For this review, take the finished solid that the model builds, in its own axes (mm). A direction names the side the tool comes from. Give positions to 0.01 mm unless a question says otherwise; leave off trailing zeros. Loops run counter-clockwise (first coordinate to the right, second up) from the corner with the lowest first, then second, coordinate; pieces in that order, holes last.
```python
from build123d import *

# Parameters (mm, degrees)
SKETCH1_W               = 60
SKETCH1_H               = 130
BOSS_EXTRUDE1_DEPTH     = 40
SKETCH2_R               = 28.25
SKETCH2_R_2             = 13.25
SKETCH2_R_3             = 17.25
SKETCH2_R_4             = 6.75
SKETCH2_R_5             = 9.5
CUT_EXTRUDE1_DEPTH      = 38
CUT_EXTRUDE9_DEPTH      = 83.006097334
CUT_EXTRUDE9_DEPTH_BACK = 83.006097334
CUT_EXTRUDE10_START     = 2
CUT_EXTRUDE10_DEPTH     = 81.006097334
CUT_EXTRUDE11_REACH     = 99.082
FILLET8_R               = 5
FILLET9_R               = 10
FILLET10_R              = 2.5
FILLET11_R              = 5


with BuildPart() as part:
    # Sketch1 → Boss-Extrude1 (new body)
    with BuildSketch(Plane(origin=(0, 0, 0), x_dir=(0, 1, 0), z_dir=(0, 0, 1))):
        Rectangle(SKETCH1_W, SKETCH1_H)
    extrude(amount=BOSS_EXTRUDE1_DEPTH)

    # Sketch2 → Cut-Extrude1 (cut)
    with BuildSketch(Plane.XY.offset(40)):
        with Locations((-35, 0)):
            Circle(SKETCH2_R)
        with Locations((37, -14.75)):
            Circle(SKETCH2_R_2)
        with Locations((12, 10.75)):
            Circle(SKETCH2_R_3)
        with Locations((56.25, 21.25)):
            Circle(SKETCH2_R_4)
        with Locations((42, 10)):
            Circle(SKETCH2_R_5)
        with BuildLine():
            Line((63, -5), (63, -25))
            ThreePointArc((63, -25), (60, -28), (57, -25))
            Line((57, -25), (57, -5))
            ThreePointArc((57, -5), (60, -2), (63, -5))
        make_face()
    extrude(amount=-CUT_EXTRUDE1_DEPTH, mode=Mode.SUBTRACT)

    # Sketch11 → Cut-Extrude9 (cut, two sides: drawn at the far end of the back side and taken through both)
    with BuildSketch(Plane(origin=(0, 0, 0), x_dir=(-1, 0, 0), z_dir=(0, 1, 0)).offset(-CUT_EXTRUDE9_DEPTH_BACK)):
        Polygon((37.662617959, 40), (-65, 40), (-65, 22.5), (-33.857500095, 22.5), (-14.42300462, 27), (19.914447088, 27), align=None)
    extrude(amount=CUT_EXTRUDE9_DEPTH + CUT_EXTRUDE9_DEPTH_BACK, mode=Mode.SUBTRACT)

    # Sketch12 → Cut-Extrude10 (cut, through all)
    with BuildSketch(Plane(origin=(0, 0, 0), x_dir=(0, 1, 0), z_dir=(0, 0, 1)).offset(CUT_EXTRUDE10_START)):
        with BuildLine():
            Line((-25.153127982, 19.113444278), (-28, 19.113444278))
            Line((-28, 19.113444278), (-28, -14.42300462))
            Line((-28, -14.42300462), (-28, -30.519259302))
            ThreePointArc((-28, -30.519259302), (-21.630520462, -23.953125349), (-12.614481333, -22.405409906))
            Line((-12.614481333, -22.405409906), (-7.568879853, -15.997641924))
            ThreePointArc((-7.568879853, -15.997641924), (-7.137176738, -6.377597635), (-1.98737408, 1.759425917))
            Line((-1.98737408, 1.759425917), (-5.735279815, 5.808065062))
            ThreePointArc((-5.735279815, 5.808065062), (-16.816114685, 10.458590364), (-25.153127982, 19.113444278))
        make_face()
    extrude(amount=CUT_EXTRUDE10_DEPTH, mode=Mode.SUBTRACT)

    # Sketch13 → Cut-Extrude11 (cut, up to next)
    with BuildSketch(Plane.XZ.offset(30), mode=Mode.PRIVATE) as cut_extrude11_sk1:
        Polygon((-15.112535459, 27), (35.351266766, 27), (6.364131369, 5), (-6.135868631, 5), align=None)
    cut_extrude11_tool1 = extrude(cut_extrude11_sk1.sketch, amount=-CUT_EXTRUDE11_REACH, mode=Mode.PRIVATE) & part.part
    add(cut_extrude11_tool1.solids().sort_by_distance((6.122185, -30, 18.210804))[0], mode=Mode.SUBTRACT)

    # Fillet8
    fillet8_edges = [part.edges().sort_by_distance(p)[0] for p in [
        (65, 30, 11.25),
        (65, -30, 11.25),
        (-65, -30, 20),
        (-65, 30, 20),
    ]]
    fillet(fillet8_edges, radius=FILLET8_R)

    # Fillet9
    # the kernel refuses this fillet: 10 mm, written as the material it adds along each edge
    with BuildSketch(Plane(origin=(33.857500095, -30, 22.5), x_dir=(1, 0, 0), z_dir=(0, 1, 0))) as fillet9_piece_1_section:
        with BuildLine():
            CenterArc((FILLET9_R * 0.114262005899, -FILLET9_R), FILLET9_R, 90, 13.036921742)
            Line((-FILLET9_R * 0.111316891577, -FILLET9_R * 0.0257750973141), (0, 0))
            Line((0, 0), (FILLET9_R * 0.114262005899, 0))
        make_face()
    fillet9_piece_1 = extrude(amount=5.234596359, mode=Mode.PRIVATE)
    fillet9_piece_1 = fillet9_piece_1 - Plane(origin=(37, -14.75, 22.477974756), x_dir=(1, 0, 0), z_dir=(0, 0, 1)) * Cylinder(13.25, 16, mode=Mode.PRIVATE)
    add(fillet9_piece_1)
    with BuildSketch(Plane(origin=(33.857500095, -4.734596359, 22.5), x_dir=(1, 0, 0), z_dir=(0, 1, 0))) as fillet9_piece_2_section:
        with BuildLine():
            CenterArc((FILLET9_R * 0.114262005899, -FILLET9_R), FILLET9_R, 90, 13.036921742)
            Line((-FILLET9_R * 0.111316891577, -FILLET9_R * 0.0257750973141), (0, 0))
            Line((0, 0), (FILLET9_R * 0.114262005899, 0))
        make_face()
    fillet9_piece_2 = extrude(amount=12.697303917, mode=Mode.PRIVATE)
    fillet9_piece_2 = fillet9_piece_2 - Plane(origin=(37, -14.75, 22.48681781), x_dir=(1, 0, 0), z_dir=(0, 0, 1)) * Cylinder(13.25, 30, mode=Mode.PRIVATE)
    fillet9_piece_2 = fillet9_piece_2 - Plane(origin=(42, 10, 22.48681781), x_dir=(1, 0, 0), z_dir=(0, 0, 1)) * Cylinder(9.5, 30, mode=Mode.PRIVATE)
    add(fillet9_piece_2)
    with BuildSketch(Plane(origin=(33.857500095, 12.037292442, 22.5), x_dir=(1, 0, 0), z_dir=(0, 1, 0))) as fillet9_piece_3_section:
        with BuildLine():
            CenterArc((FILLET9_R * 0.114262005899, -FILLET9_R), FILLET9_R, 90, 13.036921742)
            Line((-FILLET9_R * 0.111316891577, -FILLET9_R * 0.0257750973141), (0, 0))
            Line((0, 0), (FILLET9_R * 0.114262005899, 0))
        make_face()
    fillet9_piece_3 = extrude(amount=17.962707558, mode=Mode.PRIVATE)
    fillet9_piece_3 = fillet9_piece_3 - Plane(origin=(42, 10, 22.478816229), x_dir=(1, 0, 0), z_dir=(0, 0, 1)) * Cylinder(9.5, 41, mode=Mode.PRIVATE)
    add(fillet9_piece_3)
    with BuildSketch(Plane(origin=(-19.914447088, -15.708414802, 27), x_dir=(1, 0, 0), z_dir=(0, -1, 0))) as fillet9_piece_4_section:
        with BuildLine():
            CenterArc((FILLET9_R * 0.327059529607, FILLET9_R), FILLET9_R, 233.778347997, 36.221652003)
            Line((-FILLET9_R * 0.263851045123, FILLET9_R * 0.193262934611), (0, 0))
            Line((0, 0), (FILLET9_R * 0.327059529607, 0))
        make_face()
    fillet9_piece_4 = extrude(amount=14.291585198, mode=Mode.PRIVATE)
    fillet9_piece_4 = fillet9_piece_4 & Plane(origin=(-35, 0, 26.964300655), x_dir=(0.9812415105326922, -0.19278251478679478, 0), z_dir=(0, 0, -1)) * Cylinder(29.75, 42, mode=Mode.PRIVATE)
    fillet9_piece_4 = split(fillet9_piece_4, bisect_by=Plane(origin=(-19.113444278, -23.524724426, 26.964300655), z_dir=(1, 0, 0)), keep=Keep.TOP, mode=Mode.PRIVATE)
    fillet9_piece_4 = fillet9_piece_4 - Plane(origin=(-35, 0, 26.964300655), x_dir=(1, 0, 0), z_dir=(0, 0, 1)) * Cylinder(28.25, 42, mode=Mode.PRIVATE)
    add(fillet9_piece_4)
    with BuildSketch(Plane(origin=(-19.914447088, -15.708414802, 27), x_dir=(1, 0, 0), z_dir=(0, -1, 0))) as fillet9_piece_5_section:
        with BuildLine():
            CenterArc((FILLET9_R * 0.327059529607, FILLET9_R), FILLET9_R, 233.778347997, 36.221652003)
            Line((-FILLET9_R * 0.263851045123, FILLET9_R * 0.193262934611), (0, 0))
            Line((0, 0), (FILLET9_R * 0.327059529607, 0))
        make_face()
    fillet9_piece_5 = extrude(amount=14.291585198, mode=Mode.PRIVATE)
    fillet9_piece_5 = fillet9_piece_5 & Plane(origin=(-35, 0, 27.570308722), x_dir=(0.9812415105326922, -0.19278251478679478, 0), z_dir=(0, 0, -1)) * Cylinder(29.75, 42, mode=Mode.PRIVATE)
    fillet9_piece_5 = split(fillet9_piece_5, bisect_by=Plane(origin=(-19.113444278, -25.104682391, 27.570308722), z_dir=(-1, 0, 0)), keep=Keep.TOP, mode=Mode.PRIVATE)
    fillet9_piece_5 = fillet9_piece_5 - Plane(origin=(-35, 0, 27.570308722), x_dir=(1, 0, 0), z_dir=(0, 0, 1)) * Cylinder(28.25, 42, mode=Mode.PRIVATE)
    add(fillet9_piece_5)
    with BuildSketch(Plane(origin=(-19.914447088, -15.708414802, 27), x_dir=(1, 0, 0), z_dir=(0, -1, 0))) as fillet9_piece_6_section:
        with BuildLine():
            CenterArc((FILLET9_R * 0.327059529607, FILLET9_R), FILLET9_R, 233.778347997, 36.221652003)
            Line((-FILLET9_R * 0.263851045123, FILLET9_R * 0.193262934611), (0, 0))
            Line((0, 0), (FILLET9_R * 0.327059529607, 0))
        make_face()
    fillet9_piece_6 = extrude(amount=14.291585198, mode=Mode.PRIVATE)
    fillet9_piece_6 = fillet9_piece_6 - Plane(origin=(-35, 0, 27.459351012), x_dir=(0.9812415105326922, -0.19278251478679478, 0), z_dir=(0, 0, -1)) * Cylinder(29.75, 42, mode=Mode.PRIVATE)
    fillet9_piece_6 = split(fillet9_piece_6, bisect_by=Plane(origin=(-19.113444278, -26.928061773, 27.459351012), z_dir=(-1, 0, 0)), keep=Keep.TOP, mode=Mode.PRIVATE)
    fillet9_piece_6 = split(fillet9_piece_6, bisect_by=Plane(origin=(-20.316684316, -28, 27.459351012), z_dir=(0, 1, 0)), keep=Keep.TOP, mode=Mode.PRIVATE)
    add(fillet9_piece_6)
    with BuildSketch(Plane(origin=(-19.914447088, -15.708414802, 27), x_dir=(1, 0, 0), z_dir=(0, -1, 0))) as fillet9_piece_7_section:
        with BuildLine():
            CenterArc((FILLET9_R * 0.327059529607, FILLET9_R), FILLET9_R, 233.778347997, 36.221652003)
            Line((-FILLET9_R * 0.263851045123, FILLET9_R * 0.193262934611), (0, 0))
            Line((0, 0), (FILLET9_R * 0.327059529607, 0))
        make_face()
    fillet9_piece_7 = extrude(amount=14.291585198, mode=Mode.PRIVATE)
    fillet9_piece_7 = split(fillet9_piece_7, bisect_by=Plane(origin=(-19.113444278, -29, 26.965326642), z_dir=(1, 0, 0)), keep=Keep.TOP, mode=Mode.PRIVATE)
    fillet9_piece_7 = split(fillet9_piece_7, bisect_by=Plane(origin=(-18.088636338, -28, 26.965326642), z_dir=(0, -1, 0)), keep=Keep.TOP, mode=Mode.PRIVATE)
    add(fillet9_piece_7)
    with BuildSketch(Plane(origin=(-19.914447088, -15.708414802, 27), x_dir=(1, 0, 0), z_dir=(0, -1, 0))) as fillet9_piece_8_section:
        with BuildLine():
            CenterArc((FILLET9_R * 0.327059529607, FILLET9_R), FILLET9_R, 233.778347997, 36.221652003)
            Line((-FILLET9_R * 0.263851045123, FILLET9_R * 0.193262934611), (0, 0))
            Line((0, 0), (FILLET9_R * 0.327059529607, 0))
        make_face()
    fillet9_piece_8 = extrude(amount=14.291585198, mode=Mode.PRIVATE)
    fillet9_piece_8 = split(fillet9_piece_8, bisect_by=Plane(origin=(-19.113444278, -29, 27.580257853), z_dir=(-1, 0, 0)), keep=Keep.TOP, mode=Mode.PRIVATE)
    fillet9_piece_8 = split(fillet9_piece_8, bisect_by=Plane(origin=(-20.54645477, -28, 27.580257853), z_dir=(0, -1, 0)), keep=Keep.TOP, mode=Mode.PRIVATE)
    add(fillet9_piece_8)
    with BuildSketch(Plane(origin=(-19.914447088, 30, 27), x_dir=(-0.8067370653888534, 0, 0.5909105747300355), z_dir=(0, -1, 0))) as fillet9_piece_9_section:
        with BuildLine():
            CenterArc((FILLET9_R * 0.327059529607, -FILLET9_R), FILLET9_R, 90, 36.221652003)
            Line((-FILLET9_R * 0.263851045123, -FILLET9_R * 0.193262934611), (0, 0))
            Line((0, 0), (FILLET9_R * 0.327059529607, 0))
        make_face()
    fillet9_piece_9 = extrude(amount=14.291585198, mode=Mode.PRIVATE)
    fillet9_piece_9 = fillet9_piece_9 - Plane(origin=(-35, 0, 27.325753935), x_dir=(1, 0, 0), z_dir=(0, 0, 1)) * Cylinder(28.25, 42, mode=Mode.PRIVATE)
    add(fillet9_piece_9)
    # the kernel refuses this fillet: 10 mm, written as the material it takes off along each edge
    with BuildSketch(Plane(origin=(14.42300462, 32.856550147, 27), x_dir=(0.9742249026859169, 0, -0.22557889747628432), z_dir=(0, -1, 0))) as fillet9_2_piece_1:
        with BuildLine():
            CenterArc((FILLET9_R * 0.114262005899, -FILLET9_R), FILLET9_R, 90, 13.036921742)
            Line((-FILLET9_R * 0.111316891577, -FILLET9_R * 0.0257750973141), (0, 0))
            Line((0, 0), (FILLET9_R * 0.114262005899, 0))
        make_face()
    extrude(amount=7.884120565, mode=Mode.SUBTRACT)
    with BuildSketch(Plane(origin=(14.42300462, -3.472429582, 27), x_dir=(0.9742249026859169, 0, -0.22557889747628432), z_dir=(0, -1, 0))) as fillet9_2_piece_2:
        with BuildLine():
            CenterArc((FILLET9_R * 0.114262005899, -FILLET9_R), FILLET9_R, 90, 13.036921742)
            Line((-FILLET9_R * 0.111316891577, -FILLET9_R * 0.0257750973141), (0, 0))
            Line((0, 0), (FILLET9_R * 0.114262005899, 0))
        make_face()
    extrude(amount=7.226902729, mode=Mode.SUBTRACT)
    with BuildSketch(Plane(origin=(-37.662617959, 38.17648824, 40), x_dir=(0.8067370653888553, 0, -0.5909105747300331), z_dir=(0, -1, 0)), Plane(origin=(-37.662617959, -19.94775336, 40), x_dir=(0.8067370653888553, 0, -0.5909105747300331), z_dir=(0, -1, 0))) as fillet9_2_piece_3:
        with BuildLine():
            CenterArc((FILLET9_R * 0.327059529607, -FILLET9_R), FILLET9_R, 90, 36.221652003)
            Line((-FILLET9_R * 0.263851045123, -FILLET9_R * 0.193262934611), (0, 0))
            Line((0, 0), (FILLET9_R * 0.327059529607, 0))
        make_face()
    extrude(amount=18.22873488, mode=Mode.SUBTRACT)

    # Fillet10
    fillet10_edges = [part.edges().sort_by_distance(p)[0] for p in [
        (22.405409906, -12.614481333, 13.575848822),
        (15.997641924, -7.568879853, 14.317698693),
        (-1.759425917, -1.98737408, 14.5),
        (-5.808065062, -5.735279815, 14.5),
    ]]
    fillet(fillet10_edges, radius=FILLET10_R)

    # Fillet11
    fillet11_edges = [part.edges().sort_by_distance(p)[0] for p in [
        (6.364131369, -29, 5),
        (-6.135868631, -29, 5),
        (-15.112535459, -29, 27),
    ]]
    fillet(fillet11_edges, radius=FILLET11_R)


solid = part.part
```
Q1. Machinability: for faces 1 (the cylindrical face through (64, 28, 11)), 2 (the cylindrical face through (-63.223, 1.242, 17.044)), which of the approach directions +Z, -Z, +X, -X, +Y, -Y give a long, thin tool a straight path to every point of the face, cutting with its end or side? Answer none if there is none.
Answers:
face 1: +Z, -Z, +X, +Y
face 2: +Z
Q2. Consider section B-B on x = 6.5. Give the boundary of the cut face in (y, z), plus the area to 3 significant figures.
Answers:
outline: (-30, 0) - (30, 0) - (30, 27) - (27.1, 27) - (27.1, 2) - (-5.6, 2) - (-5.6, 27) - (-7.18, 27) - (-7.18, 2) - (-28, 2) - (-28, 5.34) - (-30, 5.34) - close
area: 239 mm2
Q3. For pin 1 Ø9 at (x, y) = (47, 12.5) entering from +Z; pin 2 Ø8 at (x, y) = (41, -9) entering from +Z; pin 3 Ø21 at (x, y) = (44, 12.5) entering from +Z, all flat-tipped, find the tip position at first contact; note any pin that passes through.
Answers:
pin 1: stops at z = 22.5
pin 2: stops at z = 2
pin 3: stops at z = 22.58
Q4. Consider section D-D on y = -16. Give the boundary of the cut face in (x, z).
Answers:
outline: (-65, 0) - (65, 0) - (65, 22.5) - (63, 22.5) - (63, 2) - (57, 2) - (57, 22.5) - (50.19, 22.5) - (50.19, 2) - (23.81, 2) - (23.81, 24.83) - (22.3, 25.18) - (22.3, 2) - (-9.92, 2) - (-9.92, 27) - (-11.72, 27) - (-11.72, 2) - (-58.28, 2) - (-58.28, 40) - (-65, 40) - close
Q5. Consider section A-A on y = 2. Give the boundary of the cut face in (x, z), plus the area to 3 significant figures.
Answers:
outline: (-65, 0) - (65, 0) - (65, 22.5) - (47.12, 22.5) - (47.12, 2) - (36.88, 2) - (36.88, 22.5) - (35, 22.5) arc R10 cw to (32.74, 22.76) - (26.87, 24.12) - (26.87, 2) - (-2.87, 2) - (-2.87, 27) - (-6.82, 27) - (-6.82, 2) - (-63.18, 2) - (-63.18, 40) - (-65, 40) - close
area: 1,010 mm2
Q6. Consider section C-C on x = -50.5. Give the boundary of the cut face in (y, z), plus the area to 3 significant figures.
Answers:
outline: (-30, 0) - (30, 0) - (30, 40) - (23.62, 40) - (23.62, 2) - (-23.62, 2) - (-23.62, 40) - (-30, 40) - close
area: 605 mm2
Q7. For probe 1 along Y at (x, z) = (-41, 24); probe 2 along X at (y, z) = (1.5, 17.5); probe 3 along X at (y, z) = (-9.5, 19), list the stretches that pass through material, from the lowest coordinate up.
Answers:
probe 1: y = -30 to -27.61, 27.61 to 30
probe 2: x = -65 to -63.21, -6.79 to -2.56, 26.56 to 37.76, 46.24 to 65
probe 3: x = -65 to -61.6, -8.4 to -6.81, 18.45 to 24.83, 49.17 to 57, 63 to 65
Q8. Mouldability with a two-part tool opening along X and no side actions: class faces 3 (the flat face through (54, 0, 22.5)), 4 (the cylindrical face through (60, -2, 12)), 5 (the cylindrical face through (-37.78, 29.09, 39.49)) as +X half, -X half, draft (parallel to the pull), parting line (faces both ways), or undercut.
Answers:
face 3: draft
face 4: undercut
face 5: +X half
